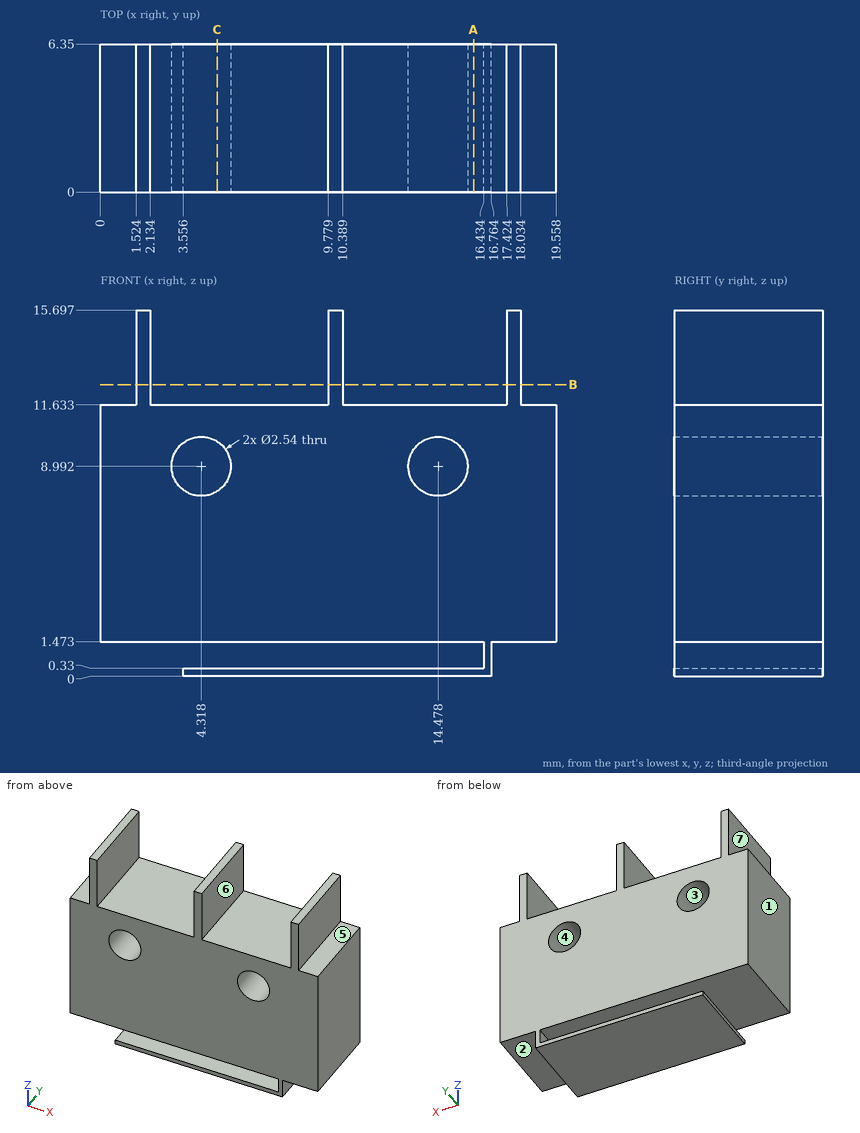
Verification items for this drawing (mm, ordinates from the low corner). A direction names the side the tool comes from. Give positions to 0.01 mm unless a question says otherwise; leave off trailing zeros. Order: outer loops, then holes, each group sorted by start corner. A loop starts at its lowest first (then second) coordinate and runs counter-clockwise, first axis right, second up. Notation, with made-up numbers: M 22.5,-34 L 63.5,-34 A35 cw 63.5,-2 Z; hole C 17.5,65.5 d4. An arc over 180 degrees is marked long. Use a Markdown table: item, result.
Item 1: Section check B-B (z = 12.5). State how many separate pieces and enclosed holes the cut face has, and give its area (3 significant figures).
Answers follow:
| item | result |
|---|---|
| separate pieces | 3 |
| enclosed holes | 0 |
| area | 11.6 mm2 |
Item 2: Tool access check on the marked faces 5, 6 and 7. Record the directions out of +Z, -Z, +X, -X, +Y, -Y that give a thin tool (end or side, any length) a straight path to the whole face; none if there is none.
Answers follow:
| item | result |
|---|---|
| face 5 | +Z, +X, +Y, -Y |
| face 6 | +Z, +Y, -Y |
| face 7 | +Z, -X, +Y, -Y |
Item 3: Depth check by flat-ended pin: P1, Ø3, axis at x = 14, y = 3, coming from the +Z side; P2, Ø1.6, axis at y = 3, z = 0.5, coming from the +X side; P3, Ø2, axis at y = 1.5, z = 13, coming from the +X side. Enter the tip coordinate at first touch or a pass-through.
Answers follow:
| item | result |
|---|---|
| P1 | stops at z = 11.63 |
| P2 | stops at x = 16.76 |
| P3 | stops at x = 18.03 |
Item 4: Material ranges on line 1 along X through (y, z) = (6, 13.75) (1 decimal); line 2 along Z through (x, y) = (9.5, 2); line 3 along Z through (x, y) = (3.75, 2.5) (1 decimal), recorded low to high.
Answers follow:
| item | result |
|---|---|
| line 1 | x = 1.5 to 2.1, 9.8 to 10.4, 17.4 to 18 |
| line 2 | z = 0 to 0.33, 1.47 to 11.63 |
| line 3 | z = 0 to 0.3, 1.5 to 7.9, 10.1 to 11.6 |
Item 5: Section check C-C (x = 5). Record the cut outline in (y, z).
Answers follow:
| item | result |
|---|---|
| outline | M 0,0 L 6.35,0 L 6.35,0.33 L 0,0.33 Z; M 0,1.47 L 6.35,1.47 L 6.35,7.92 L 0,7.92 Z; M 0,10.06 L 6.35,10.06 L 6.35,11.63 L 0,11.63 Z |
Item 6: Draft check along X on the marked faces 1, 2, 3 and 4. Enter one of: +X half, -X half, draft (parallel to the pull), parting line (faces both ways), or undercut.
Answers follow:
| item | result |
|---|---|
| face 1 | -X half |
| face 2 | draft |
| face 3 | undercut |
| face 4 | undercut |
Item 7: Section check A-A (x = 16). Record the cut outline in (y, z).
Answers follow:
| item | result |
|---|---|
| outline | M 0,0 L 6.35,0 L 6.35,0.33 L 0,0.33 Z; M 0,1.47 L 6.35,1.47 L 6.35,11.63 L 0,11.63 Z |
